Design review of the part built by this model. Coordinates are the model's own, in mm. A direction names the side the tool comes from. Round coordinates to 2 decimals unless told otherwise and drop trailing zeros. Order: outer loops, then holes, each group sorted by start corner. A loop starts at its lowest first (then second) coordinate and runs counter-clockwise, first axis right, second up. Notation, with made-up numbers: (-32.5, 49) - (-23.5, 49) arc R15 cw to (-23.5, 73) - close; hole circle Ø6 at (-33, 12.5). An arc over 180 degrees is marked (long way). Write item = value, one per line.
from build123d import *

# Parameters (mm, degrees)
SKETCH2_W           = 4
SKETCH2_H           = 1
BOSS_EXTRUDE1_DEPTH = 5


with BuildPart() as part:
    # Sketch1 → Revolve1 (revolve)
    with BuildSketch(Plane.XY, mode=Mode.PRIVATE) as revolve1_sk:
        Polygon((0, 0), (12.2, 0), (12.2, -34), (2, -34), (2, -45.5), (0, -45.5), align=None)
    revolve(revolve1_sk.sketch.rotate(Axis((0, -45.5, 0), (0, 1, 0)), 90), axis=Axis((0, -45.5, 0), (0, 1, 0)))

    # Sketch2 → Boss-Extrude1 (add)
    with BuildSketch(Plane(origin=(0, 0, 0), x_dir=(1, 0, 0), z_dir=(0, 1, 0))):
        with Locations((0, -10.5)):
            Rectangle(SKETCH2_W, SKETCH2_H)
        with Locations((0, 10.5)):
            Rectangle(SKETCH2_W, SKETCH2_H)
    extrude(amount=BOSS_EXTRUDE1_DEPTH)


solid = part.part
1) For faces 1 (the flat face through (0, 2, -11)), 2 (the cylindrical face through (2, -40, 0)), 3 (the flat face through (-2, 2.5, 10.5)), 4 (the flat face through (2, 2.5, 10.5)), list the 3-axis set-ups (+Z, -Z, +X, -X, +Y, -Y) from which the entire face can be reached by the end or side of a thin tool; tool diameter is ignored.
Findings:
face_1 = -Z, +X, -X, +Y
face_2 = -Y
face_3 = +Z, -Z, -X, +Y
face_4 = +Z, -Z, +X, +Y
2) Clearance check with flat-ended pins moving along their axes: pin 1 Ø3 at (x, y) = (1, 2.5) entering from +Z; pin 2 Ø10 at (x, z) = (-4.5, -4.5) entering from +Y; pin 3 Ø4 at (y, z) = (-36.5, -3.5) entering from -X; pin 4 Ø6 at (x, y) = (-5.5, -37.5) entering from +Z. State where each tip first meets the part, or that it passes through.
Findings:
pin_1 = 11
pin_2 = 0
pin_3 = -1.32
pin_4 = through
3) The part is to be moulded in two halves that separate along Z. For faces 5 (the flat face through (0, 2, 10)), 6 (the flat face through (0, 2, 11)), 7 (the cylindrical face through (7.4, -17.2, 9.7)), 8 (the flat face through (-2, 2.5, -10.5)), say which applies: released by +Z, released by -Z, zero draft, split by the parting line, or undercut.
Findings:
face_5 = undercut
face_6 = released by +Z
face_7 = split by the parting line
face_8 = zero draft
4) To check wall thickness, follow L1, parallel to Y at x = 3, z = 8.5; L2, parallel to Y at x = 0.75, z = -0.5; L3, parallel to X at y = -27, z = 0.25. State the ranges of each line that lie inside material, in increasing order. Write a range as from..to.
Findings:
L1 = -34..0
L2 = -45.5..0
L3 = -12.2..12.2
5) We need section D-D on y = -11.5. Write out the cut boundary in (x, z).
Findings:
outline = circle Ø24.4 at (0, 0)
6) We need section A-A on x = 0. Write out the cut boundary in (y, z), and give its area (3 significant figures).
Findings:
outline = (-45.5, -2) - (-34, -2) - (-34, -12.2) - (0, -12.2) - (0, -11) - (5, -11) - (5, -10) - (0, -10) - (0, 10) - (5, 10) - (5, 11) - (0, 11) - (0, 12.2) - (-34, 12.2) - (-34, 2) - (-45.5, 2) - close
area = 886 mm^2
7) We need section B-B on z = 0. Write out the cut boundary in (x, y).
Findings:
outline = (-12.2, -34) - (-2, -34) - (-2, -45.5) - (2, -45.5) - (2, -34) - (12.2, -34) - (12.2, 0) - (-12.2, 0) - close
8) We need section C-C on y = -38. Write out the cut boundary in (x, z).
Findings:
outline = circle Ø4 at (0, 0)
